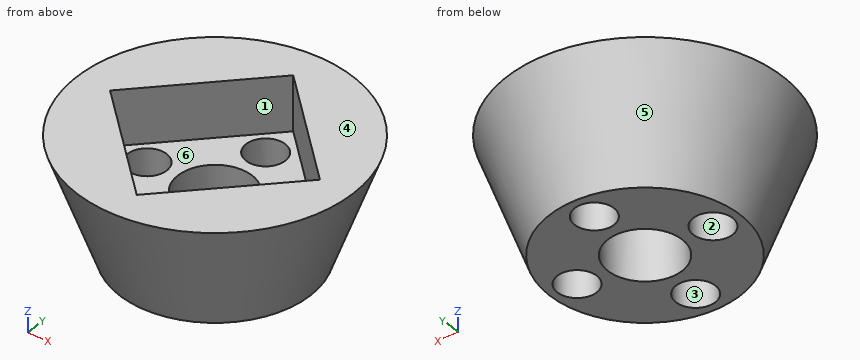
from build123d import *

# Parameters (mm, degrees)
GEARFACEPROFILE_R           = 12.2
GEARFACEEXTRUDE_DEPTH       = 15
GEARFACEEXTRUDE_TAPER       = -20
CENTERHOLEPROFILE_R         = 4.75
CENTERHOLECUT_DEPTH         = 16.0000001
SCREWHOLEPROFILE_R          = 2.52
SCREWHOLECUT_DEPTH          = 16.0000001
SHAFTCOLLARDOCKINGCUT_DEPTH = 7


with BuildPart() as part:
    # GearFaceProfile → GearFaceExtrude (new body)
    with BuildSketch(Plane.XY):
        Circle(GEARFACEPROFILE_R)
    extrude(amount=GEARFACEEXTRUDE_DEPTH, taper=GEARFACEEXTRUDE_TAPER)

    # CenterHoleProfile → CenterHoleCut (cut, through all)
    with BuildSketch(Plane(origin=(0, 0, 0), x_dir=(-1, 0, 0), z_dir=(0, 0, -1))):
        Circle(CENTERHOLEPROFILE_R)
    extrude(amount=-CENTERHOLECUT_DEPTH, mode=Mode.SUBTRACT)

    # ScrewHoleProfile → ScrewHoleCut (cut, through all)
    with BuildSketch(Plane(origin=(0, 0, 0), x_dir=(-1, 0, 0), z_dir=(0, 0, -1))):
        with Locations((0, 8.7)):
            Circle(SCREWHOLEPROFILE_R)
        with Locations((8.7, 0)):
            Circle(SCREWHOLEPROFILE_R)
        with Locations((0, -8.7)):
            Circle(SCREWHOLEPROFILE_R)
        with Locations((-8.7, 0)):
            Circle(SCREWHOLEPROFILE_R)
    extrude(amount=-SCREWHOLECUT_DEPTH, mode=Mode.SUBTRACT)

    # ShaftCollarAttachmentProfile → ShaftCollarDockingCut (cut)
    with BuildSketch(Plane.XY.offset(15)):
        Polygon((0, 13.435028843), (13.435028843, 0), (0, -13.435028843), (-13.435028843, 0), align=None)
    extrude(amount=-SHAFTCOLLARDOCKINGCUT_DEPTH, mode=Mode.SUBTRACT)


solid = part.part
Here's how the part is built. I have some questions about the finished solid (model axes, mm). Face numbers are marked on the shaded views. A direction names the side the tool comes from. Round coordinates to 2 decimals unless told otherwise and drop trailing zeros. Loops run counter-clockwise (first coordinate to the right, second up) from the corner with the lowest first, then second, coordinate; pieces in that order, holes last. Notation, with made-up numbers: (-4.5, 22) -> (38.5, 22) arc R32 ccw to (38.5, 52) -> close; hole circle Ø8 at (9, 62.25). An arc over 180 degrees is marked (long way). Write each question's results on one line, items separated by ' | '.
(1) For the marked faces 1 and 2, which set-ups out of +Z, -Z, +X, -X, +Y, -Y let a thin tool reach every point of the face, with its end or its side?
Worked answers:
face 1: +Z | face 2: +Z, -Z
(2) If we section it at B-B, the plane y = -2: Give the number of separate pieces and of enclosed holes in the cut face, then the cut area to 3 significant figures.
Worked answers:
separate pieces: 4 | enclosed holes: 0 | area: 166 mm2
(3) We'd pull the mould along X, two halves only. Please class the marked faces 3, 4, 5 and 6: released by +X, released by -X, zero draft, split by the parting line, or undercut.
Worked answers:
face 3: undercut | face 4: zero draft | face 5: split by the parting line | face 6: undercut
(4) If I drill on L1, parallel to Y at x = 0, z = 5; L2, parallel to Y at x = 0, z = 4.5; L3, parallel to X at y = -6.5, z = 7.75, over which ranges is the centre line in solid material (lowest first)?
Worked answers:
L1: -14.02 to -11.22, -6.18 to -4.75, 4.75 to 6.18, 11.22 to 14.02 | L2: -13.84 to -11.22, -6.18 to -4.75, 4.75 to 6.18, 11.22 to 13.84 | L3: -13.54 to -1.23, 1.23 to 13.54
(5) If we section it at C-C, the plane z = 6: List the corners of the cut face in (x, y) for me.
Worked answers:
outline: circle Ø28.77 at (0, 0); hole circle Ø5.04 at (-8.7, 0); hole circle Ø9.5 at (0, 0); hole circle Ø5.04 at (0, -8.7); hole circle Ø5.04 at (0, 8.7); hole circle Ø5.04 at (8.7, 0)
(6) If we section it at A-A, the plane z = 10.5: List the corners of the cut face in (x, y) for me, then the cut area to 3 significant figures.
Worked answers:
outline: circle Ø32.04 at (0, 0); hole (-13.44, 0) -> (0, -13.44) -> (13.44, 0) -> (0, 13.44) -> close | area: 445 mm2
(7) For P1, Ø3, axis at y = 6, z = 7.5, coming from the +X side; P2, Ø3, axis at x = 7.5, z = 3.5, coming from the -Y side; P3, Ø1, axis at y = 8, z = 11.5, coming from the -X side, each with a flat end and sliding along its axis, tell me the tip position at first contact or that it passes through.
Worked answers:
P1: x = 14.5 | P2: y = -12.28 | P3: x = -14.64
